from build123d import *

# Parameters (mm, degrees)
ESBO_O1_R                = 27.5
ESBO_O1_R_2              = 5.5
ESBO_O1_R_3              = 1.25
RESSALTO_EXTRUS_O1_DEPTH = 2
FILETE1_R                = 17.5


with BuildPart() as part:
    # Esboço1 → Ressalto-extrusão1 (new body)
    with BuildSketch(Plane.XY):
        with BuildLine():
            Line((-165, 17.5), (-165, -17.5))
            Line((-165, -17.5), (-51.659945799, -17.5))
            ThreePointArc((-51.659945799, -17.5), (-35.617722101, -20.143405329), (-21.271742388, -27.794117647))
            ThreePointArc((-21.271742388, -27.794117647), (35, 0), (-21.271742388, 27.794117647))
            ThreePointArc((-21.271742388, 27.794117647), (-35.617722101, 20.143405329), (-51.659945799, 17.5))
            Line((-51.659945799, 17.5), (-165, 17.5))
        make_face()
        Circle(ESBO_O1_R, mode=Mode.SUBTRACT)
        with Locations((-147.5, 0)):
            Circle(ESBO_O1_R_2, mode=Mode.SUBTRACT)
        with Locations((-147.5, 11)):
            Circle(ESBO_O1_R_3, mode=Mode.SUBTRACT)
        with Locations((-139.721825407, 7.778174593)):
            Circle(ESBO_O1_R_3, mode=Mode.SUBTRACT)
        with Locations((-136.5, 0)):
            Circle(ESBO_O1_R_3, mode=Mode.SUBTRACT)
        with Locations((-139.721825407, -7.778174593)):
            Circle(ESBO_O1_R_3, mode=Mode.SUBTRACT)
        with Locations((-147.5, -11)):
            Circle(ESBO_O1_R_3, mode=Mode.SUBTRACT)
        with Locations((-155.278174593, -7.778174593)):
            Circle(ESBO_O1_R_3, mode=Mode.SUBTRACT)
        with Locations((-158.5, 0)):
            Circle(ESBO_O1_R_3, mode=Mode.SUBTRACT)
        with Locations((-155.278174593, 7.778174593)):
            Circle(ESBO_O1_R_3, mode=Mode.SUBTRACT)
        with Locations((31.5, 0)):
            Circle(ESBO_O1_R_3, mode=Mode.SUBTRACT)
        with Locations((-57.5, 12.5)):
            Circle(ESBO_O1_R_3, mode=Mode.SUBTRACT)
        with Locations((-102.5, 12.5)):
            Circle(ESBO_O1_R_3, mode=Mode.SUBTRACT)
        with Locations((-102.5, -12.5)):
            Circle(ESBO_O1_R_3, mode=Mode.SUBTRACT)
        with Locations((-57.5, -12.5)):
            Circle(ESBO_O1_R_3, mode=Mode.SUBTRACT)
    extrude(amount=RESSALTO_EXTRUS_O1_DEPTH)

    # Filete1
    filete1_edges = [part.edges().sort_by_distance(p)[0] for p in [
        (-165, -17.5, 1),
        (-165, 17.5, 1),
    ]]
    fillet(filete1_edges, radius=FILETE1_R - 0.0001)  # a hair under: the kernel refuses the full size


solid = part.part
Verification items for the finished model (mm, model axes). Coordinates: 2 decimals unless noted, no trailing zeros. Order: outer loops, then holes, each group sorted by start corner. A loop starts at its lowest first (then second) coordinate and runs counter-clockwise, first axis right, second up. Notation, with made-up numbers: M -40,-35 L 4,-35 A6 ccw 4,-29 Z; hole C 59.25,-14 d10. An arc over 180 degrees is marked long. One line per item, written item: value. Start each with the question number.
Item 1: Sectioned sample at D-D on x = -115. Record the cut outline in (y, z).
Item 2: Sectioned sample at B-B on x = -2.5. Record the cut outline in (y, z), then the cut area to 3 significant figures.
Item 3: Sectioned sample at A-A on y = 24. Record the cut outline in (x, z), then the cut area to 3 significant figures.
Item 4: Sectioned sample at C-C on z = 0.8. Give the number of separate pieces and of enclosed holes in the cut face, then the cut area to 3 significant figures.
Item 5: Mould release check, pull along X, two halves, no side actions. Record for faces 1 (the cylindrical face through (-5.961, -26.846, 0.986)), 2 (the cylindrical face through (-160.01, 12.24, 1.01)), 3 (the cylindrical face through (34.983, -1.09, 0.986)): pulls with the +X half, pulls with the -X half, needs draft (parallel to the pull), parting line crosses it, or undercut.
Item 6: Depth check by flat-ended pin: P1, Ø0.6, axis at x = -102, z = 1, coming from the +Y side. Enter the tip coordinate at first touch or a pass-through.
Item 7: Thickness scan on probe 1 along Y at (x, z) = (-102.5, 1); probe 2 along X at (y, z) = (3, 1.35); probe 3 along X at (y, z) = (10.5, 0.7). Record the ranges inside material, lowest first.
Calculated:
1. outline: M -17.5,0 L 17.5,0 L 17.5,2 L -17.5,2 Z
2. outline: M -34.91,0 L -27.39,0 L -27.39,2 L -34.91,2 Z; M 27.39,0 L 34.91,0 L 34.91,2 L 27.39,2 Z
2. area: 30.1 mm^2
3. outline: M -27.01,0 L -13.43,0 L -13.43,2 L -27.01,2 Z; M 13.43,0 L 25.48,0 L 25.48,2 L 13.43,2 Z
3. area: 51.3 mm^2
4. separate pieces: 1
4. enclosed holes: 15
4. area: 5,880 mm^2
5. face 1: undercut
5. face 2: pulls with the -X half
5. face 3: parting line crosses it
6. P1: y = 17.5
7. probe 1: -17.5 to -13.75, -11.25 to 11.25, 13.75 to 17.5
7. probe 2: -164.74 to -152.11, -142.89 to -27.34, 27.34 to 34.87
7. probe 3: -161.5 to -148.65, -146.35 to -25.42, 25.42 to 33.39
